Model file for the job. Use its own axes, mm. A direction names the side the tool comes from. Coordinates: 2 decimals unless noted, no trailing zeros. Write each loop counter-clockwise with the first axis right and the second up, starting at its lowest first coordinate (ties: lowest second). Pieces come first, ordered by that corner, then holes. Notation, with made-up numbers: M 78,65.5 L 92,65.5 A24 ccw 92,76.5 Z; hole C -4,3 d10. An arc over 180 degrees is marked long. Put each result on its own line as item: value. Start each with the question number.
Q1. Cut at B-B (z = -5.5). Write the cut outline in (x, y), then the cut area to 3 significant figures.
Q2. Drop flat-ended pins along their axis: pin 1 (3 mm diameter, centred on x = -105.5, y = -8, fed in from -Z); pin 2 (5 mm diameter, centred on x = 103.5, z = 0, fed in from -Y); pin 3 (3 mm diameter, centred on x = -106.5, y = -9, fed in from +Z). Give the stop position or say it passes through.
Q3. Which spindle directions (+Z, -Z, +X, -X, +Y, -Y) get a long thin tool onto all of the face, cutting with end or side? Do faces 1 (the flat face through (105, -15, 0)), 2 (the flat face through (105, -5, 0)), 3 (the flat face through (-105, -15, 0)). Say none if no direction does.
Q4. Cut at C-C (y = -17.75). Write the cut outline in (x, z).
Q5. Cut at A-A (y = -8). Write the cut outline in (x, z), then the cut area to 3 significant figures.
Q6. Drill centre lines: line 1 along X through (y, z) = (-11, 13); line 2 along Y through (x, z) = (-101, 3.75). Where is each one in solid material? Low to high.
```python
from build123d import *

# Parameters (mm, degrees)
F0_W     = 200
F0_H     = 30
F1_DEPTH = 20
F2_W     = 10
F2_H     = 20
F3_DEPTH = 10


with BuildPart() as f1:
    # F0 (on Front) → F1 (new body)
    with BuildSketch(Plane.XZ):
        Rectangle(F0_W, F0_H)
    extrude(amount=F1_DEPTH)

    # F2 (on face) → F3 (join)
    with BuildSketch(Plane(origin=(-100, 0, 0), x_dir=(0, -1, 0), z_dir=(-1, 0, 0))):
        with Locations((10, 0)):
            Rectangle(F2_W, F2_H)
    extrude(amount=F3_DEPTH)

    # F4: F1 across plane


with BuildPart() as f1_1:
    add(f1.part)
    add(f1.part.mirror(Plane.YZ))


solid = f1_1.part
```
Computed values:
1. outline: M -110,-15 L -100,-15 L -100,-20 L 100,-20 L 100,-15 L 110,-15 L 110,-5 L 100,-5 L 100,0 L -100,0 L -100,-5 L -110,-5 Z
1. area: 4,200 mm2
2. pin 1: z = -10
2. pin 2: y = -15
2. pin 3: z = 10
3. face 1: +Z, -Z, +X, -Y
3. face 2: +Z, -Z, +X, +Y
3. face 3: +Z, -Z, -X, -Y
4. outline: M -100,-15 L 100,-15 L 100,15 L -100,15 Z
5. outline: M -110,-10 L -100,-10 L -100,-15 L 100,-15 L 100,-10 L 110,-10 L 110,10 L 100,10 L 100,15 L -100,15 L -100,10 L -110,10 Z
5. area: 6,400 mm2
6. line 1: -100 to 100
6. line 2: -15 to -5
